For this review, take the finished solid that the model builds, in its own axes (mm). Round coordinates to 2 decimals unless told otherwise and drop trailing zeros. Write each loop counter-clockwise with the first axis right and the second up, starting at its lowest first coordinate (ties: lowest second). Pieces come first, ordered by that corner, then holes.
from build123d import *

# Parameters (mm, degrees)
BOSS_EXTRUDE1_DEPTH                      = 3
MIRROR1_AT_THE_SECOND_PLANE_COPY_1_DEPTH = 3


with BuildPart() as part:
    # Sketch1 → Boss-Extrude1 (new body)
    with BuildSketch(Plane(origin=(0, 0, 0), x_dir=(1, 0, 0), z_dir=(0, 1, 0))):
        Polygon((-76, -73), (-59.111111111, -73), (-59.111111111, -76), (-42.222222222, -76), (-42.222222222, -73), (-25.333333333, -73), (-25.333333333, -76), (-8.444444444, -76), (-8.444444444, -73), (0, -73), (0, 0), (-76, 0), (-76, -8.444444444), (-73, -8.444444444), (-73, -25.333333333), (-76, -25.333333333), (-76, -42.222222222), (-73, -42.222222222), (-73, -59.111111111), (-76, -59.111111111), align=None)
    boss_extrude1 = extrude(amount=BOSS_EXTRUDE1_DEPTH)



with BuildPart() as mirror1_1:
    # Mirror1: Boss-Extrude1 across plane
    add(boss_extrude1.mirror(Plane(origin=(0, 0, 0), x_dir=(0, 0, 1), z_dir=(1, 0, 0))))


with BuildPart() as part_1:
    add(part.part)

    add(mirror1_1.part)  # Mirror1 at the second plane merges Mirror1_1
    # Mirror1 at the second plane: Boss-Extrude1 across plane
    add(boss_extrude1.mirror(Plane.XY))

    # Mirror1 at the second plane copy 1 sketc → Mirror1 at the second plane copy 1 (add)
    with BuildSketch(Plane(origin=(0, 0, 0), x_dir=(-1, 0, 0), z_dir=(0, 1, 0))):
        Polygon((-76, -73), (-59.111111111, -73), (-59.111111111, -76), (-42.222222222, -76), (-42.222222222, -73), (-25.333333333, -73), (-25.333333333, -76), (-8.444444444, -76), (-8.444444444, -73), (0, -73), (0, 0), (-76, 0), (-76, -8.444444444), (-73, -8.444444444), (-73, -25.333333333), (-76, -25.333333333), (-76, -42.222222222), (-73, -42.222222222), (-73, -59.111111111), (-76, -59.111111111), align=None)
    extrude(amount=MIRROR1_AT_THE_SECOND_PLANE_COPY_1_DEPTH)


solid = part_1.part
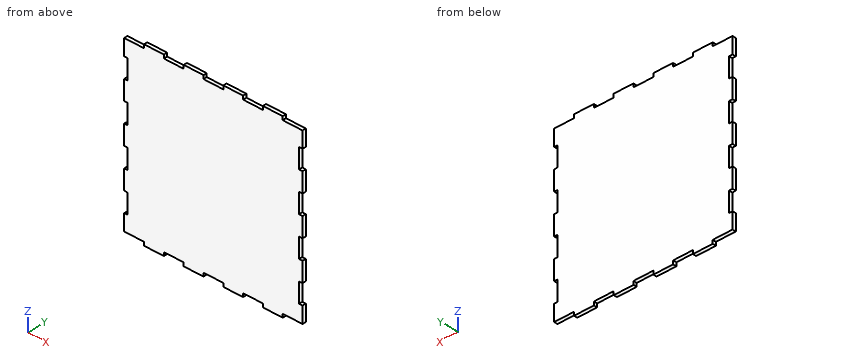
(1) For pin 1 Ø0.9 at (x, y) = (-75, 1) entering from -Z; pin 2 Ø1.5 at (x, y) = (71, 1.5) entering from +Z; pin 3 Ø0.9 at (y, z) = (1, -74) entering from +X, all flat-tipped, find the tip position at first contact; note any pin that passes through.
Geometry check:
pin 1: stops at z = -73
pin 2: stops at z = 73
pin 3: stops at x = 59.11
(2) For line 1 along X through (y, z) = (2.55, -58), list the stretches that pass through material, from the lowest coordinate up.
Geometry check:
line 1: x = -73 to 73
(3) We need section A-A, the plane x = 66.5. Give the boundary of the cut face in (y, z).
Geometry check:
outline: (0, -73) - (3, -73) - (3, 73) - (0, 73) - close
(4) We need section B-B, the plane z = -47.5. Give the boundary of the cut face in (x, y), and give its area (3 significant figures).
Geometry check:
outline: (-73, 0) - (73, 0) - (73, 3) - (-73, 3) - close
area: 438 mm2
